The model under review builds one solid part; all positions refer to its coordinate system, in mm. Face numbers are marked on the shaded views. A direction names the side the tool comes from. Coordinates: 2 decimals unless noted, no trailing zeros. Loops run counter-clockwise (first coordinate to the right, second up) from the corner with the lowest first, then second, coordinate; pieces in that order, holes last. Notation, with made-up numbers: (-14.5, 47.25) - (3.5, 47.25) arc R16 ccw to (3.5, 78.25) - close; hole circle Ø6 at (37.5, 15.25). An arc over 180 degrees is marked (long way). Use a Markdown table: item, result. Add a question column.
1) To check wall thickness, follow L1, parallel to X at y = 0, z = 12.6; L2, parallel to X at y = 0, z = 7; L3, parallel to Y at x = -6.4, z = 0.7. State the ranges of each line that lie inside material, in increasing order. Write a range as [from, to].
2) Clearance check with flat-ended pins moving along their axes: pin 1 (2.5 mm diameter, centred on x = -18, y = -0.5, fed in from +Z); pin 2 (3 mm diameter, centred on x = 18.5, y = -1, fed in from +Z); pin 3 (2.5 mm diameter, centred on x = 1, z = 14.5, fed in from +Y). State where each tip first meets the part, or that it passes through.
3) For the marked faces 4, 5 and 6, list the 3-axis set-ups (+Z, -Z, +X, -X, +Y, -Y) from which the entire face can be reached by the end or side of a thin tool; tool diameter is ignored.
4) Add section C-C, the plane z = 11.5. Give the boundary of the cut face in (x, y), and give its area (3 significant figures).
5) The part is to be moulded in two halves that separate along Y. For the marked faces 1, 2 and 3, say which applies: pulls with the +Y half, pulls with the -Y half, needs draft (parallel to the pull), parting line crosses it, or undercut.
6) Add section A-A, the plane y = -14.5. Give the boundary of the cut face in (x, z).
7) Add section D-D, the plane z = 15.25. Give the boundary of the cut face in (x, y), and give its area (3 significant figures).
8) Add section B-B, the plane x = -6.4. Give the number of separate pieces and of enclosed holes in the cut face, and give its area (3 significant figures).
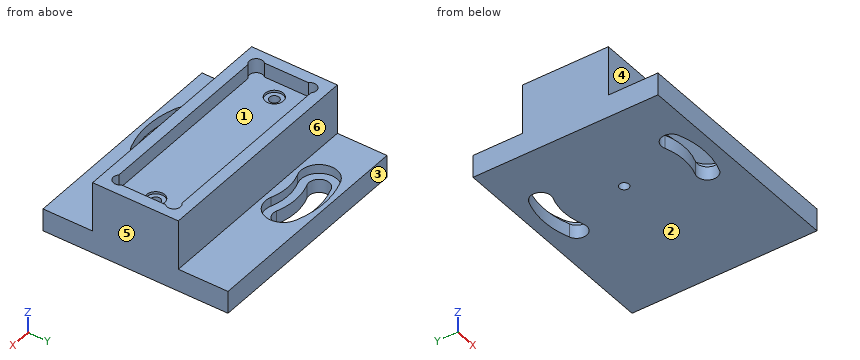
Autodesk Inventor part; units mm, degrees
ref_plane "YZ Plane" through (0, 0, 0) normal (1, 0, 0) x (0, 1, 0)
ref_plane "XZ Plane" through (0, 0, 0) normal (0, 1, 0) x (-1, 0, 0)
ref_plane "XY Plane" through (0, 0, 0) normal (0, 0, 1) x (1, 0, 0)
sketch "Sketch1" plane through (0, 0, 0) normal (0, 0, 1) x (1, 0, 0)
  line L0 (-24.4, -9.5) -> (24.4, -9.5)
  line L1 (24.4, -9.5) -> (24.4, 9.5)
  line L2 (24.4, 9.5) -> (-24.4, 9.5)
  line L3 (-24.4, 9.5) -> (-24.4, -9.5)
  line L4 (-24.4, -9.5) -> (24.4, 9.5) construction
  line L5 (24.4, -9.5) -> (-24.4, 9.5) construction
  point P0 (0, 0)
  dimension "LENGTH" = 48.8
  dimension "WIDTH" = 19
extrude "Extrusion1" add sketch "Sketch1" along normal blind 12.85
sketch "Sketch2" plane through (0, 0, 12.85) normal (0, 0, 1) x (1, 0, 0)
  point P0 (0, 0)
  point P1 (-18.2, 0)
  point P2 (18.2, 0)
  dimension "d11" = 0
  dimension "d12" = 0
  dimension "d13" = 36.4
  dimension "d14" = 18.2
hole "Hole1" at (-18.2, 0, 12.85) at (18.2, 0, 12.85) direction (0, 0, -1) diameter 2.1565 depth 8.87
sketch "Sketch3" plane through (0, 0, 12.85) normal (0, 0, 1) x (1, 0, 0)
  point P0 (0, 0)
  point P1 (0, 0)
  dimension "d22" = 0
  dimension "d23" = 0
hole "Hole2" [suppressed]
sketch "Sketch4" plane through (0, 0, 0) normal (0, 0, -1) x (-1, 0, 0)
  line L0 (5.5, 0) -> (4.5, 0) construction
  line L1 (5.5, 1.05) -> (4.5, 1.05)
  line L2 (4.5, -1.05) -> (5.5, -1.05)
  arc A0 (5.5, -1.05) -> (5.5, 1.05) centre (5.5, 0) ccw
  arc A1 (4.5, 1.05) -> (4.5, -1.05) centre (4.5, 0) ccw
  point P0 (0, 0)
  point P1 (-5, 0)
  point P2 (5, 0)
  dimension "d24" = 1
  dimension "d25" = 0
  dimension "d26" = 0
  dimension "d27" = 10
  dimension "d28" = 5
  dimension "d29" = 1.05
hole "Hole3" [suppressed]
extrude "Extrusion2" [suppressed]
sketch "Sketch5" plane through (0, 0, 0) normal (0, 0, 1) x (1, 0, 0)
  line L0 (-24.4, -20.5) -> (24.4, -20.5)
  line L1 (24.4, -20.5) -> (24.4, 20.5)
  line L2 (24.4, 20.5) -> (-24.4, 20.5)
  line L3 (-24.4, 20.5) -> (-24.4, -20.5)
  line L4 (-24.4, -20.5) -> (24.4, 20.5) construction
  line L5 (24.4, -20.5) -> (-24.4, 20.5) construction
  point P0 (0, 0)
  dimension "d39" = 48.8
  dimension "d40" = 41
extrude "Extrusion3" add sketch "Sketch5" along normal blind 5
sketch "Sketch7" plane through (0, 0, 12.85) normal (0, 0, 1) x (1, 0, 0)
  circle A0 centre (18.2, 0) radius 1.0782
  circle A1 centre (-18.2, 0) radius 1.0782
  point P0 (0, 0)
  dimension "d54" = 0
  dimension "d55" = 0
  dimension "d56" = 0
  dimension "d57" = 0
hole "Hole5" at (18.2, 0, 12.85) at (-18.2, 0, 12.85) direction (0, 0, -1) diameter 4 depth 0.5
sketch "Sketch8" plane through (0, 0, 0) normal (0, 0, -1) x (-1, 0, 0)
  line L0 (0, 5.5) -> (0, 4.5) construction
  line L1 (-1.05, 5.5) -> (-1.05, 4.5)
  line L2 (1.05, 4.5) -> (1.05, 5.5)
  arc A0 (1.05, 5.5) -> (-1.05, 5.5) centre (0, 5.5) ccw
  arc A1 (-1.05, 4.5) -> (1.05, 4.5) centre (0, 4.5) ccw
  point P0 (0, 0)
  point P1 (0, -5)
  point P2 (0, 5)
  dimension "d77" = 1
  dimension "d78" = 1.05
  dimension "d79" = 10
  dimension "d80" = 0
  dimension "d81" = 0
  dimension "d82" = 5
hole "Hole6" [suppressed]
extrude "Extrusion4" [suppressed]
sketch "Sketch10" plane through (0, 0, 12.85) normal (0, 0, 1) x (1, 0, 0)
  line L0 (-24.4, -9.5) -> (24.4, -9.5)
  line L1 (24.4, -9.5) -> (24.4, 9.5)
  line L2 (24.4, 9.5) -> (-24.4, 9.5)
  line L3 (-24.4, 9.5) -> (-24.4, -9.5)
  line L4 (-24.4, -9.5) -> (24.4, 9.5) construction
  line L5 (24.4, -9.5) -> (-24.4, 9.5) construction
  line L6 (21.9, -7) -> (-21.9, -7)
  line L7 (-21.9, -7) -> (-21.9, 7)
  line L8 (-21.9, 7) -> (21.9, 7)
  line L9 (21.9, 7) -> (21.9, -7)
  line L10 (21.9, -7) -> (-21.9, 7) construction
  line L11 (-21.9, -7) -> (21.9, 7) construction
  circle A0 centre (-20.8393, 5.9393) radius 1.5
  circle A1 centre (-20.8393, -5.9393) radius 1.5
  circle A2 centre (20.8393, 5.9393) radius 1.5
  circle A3 centre (20.8393, -5.9393) radius 1.5
  line L12 (20.8393, 5.9393) -> (21.9, 7)
  line L13 (21.9, -7) -> (20.8393, -5.9393)
  line L14 (-20.8393, 5.9393) -> (-21.9, 7)
  line L15 (-20.8393, -5.9393) -> (-21.9, -7)
  point P0 (0, 0)
  point P1 (21.9, -4.8787)
  point P2 (19.7787, -7)
  point P3 (-19.7787, -7)
  point P4 (-21.9, -4.8787)
  point P5 (-21.9, 4.8787)
  point P6 (-19.7787, 7)
  point P7 (19.7787, 7)
  point P8 (21.9, 4.8787)
  dimension "d106" = 3
  dimension "d110" = 3
  dimension "d111" = 3
  dimension "d112" = 3
  dimension "d97" = 48.8
  dimension "d98" = 19
  dimension "d99" = 43.8
  dimension "d100" = 14
  dimension "d107" = 45
  dimension "d108" = 45
  dimension "d109" = 45
extrude "Extrusion6" add sketch "Sketch10" along normal blind 3.2
chamfer "Chamfer5" [suppressed]
sketch "Sketch12" plane through (0, 0, 5) normal (0, 0, 1) x (1, 0, 0)
  arc A0 (7.9961, 15.4962) -> (-8.004, 14.5013) centre (9.4196, -136.543) ccw construction
  arc A1 (7.9587, 19.496) -> (-8.4624, 18.4749) centre (9.4196, -136.543) ccw
  arc A2 (8.0336, 11.4964) -> (-7.5457, 10.5276) centre (9.4196, -136.543) ccw
  arc A3 (8.0336, 11.4964) -> (7.9587, 19.496) centre (7.9961, 15.4962) ccw
  arc A4 (-8.4624, 18.4749) -> (-7.5457, 10.5276) centre (-8.004, 14.5013) ccw
  line L0 (24.4, 2.961) -> (24.4, -2.961)
  line L1 (24.4, 0) -> (-24.4, 0)
  line L2 (-24.4, 8.5) -> (-24.4, -8.5)
  arc A5 (7.9961, 15.4962) -> (-8.004, 14.5013) centre (9.4196, -136.543) ccw construction
  arc A6 (7.9751, 17.7461) -> (-8.2619, 16.7364) centre (9.4196, -136.543) ccw
  arc A7 (8.0172, 13.2463) -> (-7.7462, 12.2661) centre (9.4196, -136.543) ccw
  arc A8 (8.0172, 13.2463) -> (7.9751, 17.7461) centre (7.9961, 15.4962) ccw
  arc A9 (-8.2619, 16.7364) -> (-7.7462, 12.2661) centre (-8.004, 14.5013) ccw
  arc A10 (-8.004, -14.5013) -> (7.9961, -15.4962) centre (9.4196, 136.543) ccw construction
  arc A11 (-8.4624, -18.4749) -> (7.9587, -19.496) centre (9.4196, 136.543) ccw
  arc A12 (-7.5457, -10.5276) -> (8.0336, -11.4964) centre (9.4196, 136.543) ccw
  arc A13 (7.9587, -19.496) -> (8.0336, -11.4964) centre (7.9961, -15.4962) ccw
  arc A14 (-7.5457, -10.5276) -> (-8.4624, -18.4749) centre (-8.004, -14.5013) ccw
  arc A15 (-8.004, -14.5013) -> (7.9961, -15.4962) centre (9.4196, 136.543) ccw construction
  arc A16 (-8.2619, -16.7364) -> (7.9751, -17.7461) centre (9.4196, 136.543) ccw
  arc A17 (-7.7462, -12.2661) -> (8.0172, -13.2463) centre (9.4196, 136.543) ccw
  arc A18 (7.9751, -17.7461) -> (8.0172, -13.2463) centre (7.9961, -15.4962) ccw
  arc A19 (-7.7462, -12.2661) -> (-8.2619, -16.7364) centre (-8.004, -14.5013) ccw
  point P0 (0, 0)
  point P1 (-8.004, 12.753)
  point P2 (7.9961, 17.2527)
  point P3 (-6.4165, 14.3405)
  point P4 (9.5836, 18.8402)
  point P5 (-8.004, -12.753)
  point P6 (7.9961, -17.2527)
  point P7 (9.5836, -18.8402)
  point P8 (-6.4165, -14.3405)
  dimension "d118" = 8
  dimension "d122" = 4.5
extrude "Extrusion12" [suppressed]
extrude "Extrusion13" [suppressed]
sketch "Sketch14" plane through (0, 0, 0) normal (0, 0, -1) x (-1, 0, 0)
  point P0 (0, 0)
  point P1 (6.4, 0)
hole "Hole7" at (-6.4, 0, 0) direction (0, 0, 1) diameter 2.1 depth 2.1
sketch "Sketch15" plane through (0, 0, 0) normal (0, 0, -1) x (-1, 0, 0)
  circle A0 centre (6.4, 0) radius 1.05
  circle A1 centre (6.4, 0) radius 19.5
  circle A2 centre (6.4, 0) radius 11.5
  circle A3 centre (6.4, 0) radius 17.75
  circle A4 centre (6.4, 0) radius 13.25
  line L0 (-24.4, 9.5) -> (24.4, 9.5)
  line L1 (24.4, 9.5) -> (-24.4, 9.5)
  line L2 (-24.4, -20.5) -> (-24.4, 20.5)
  line L3 (24.4, -9.5) -> (-24.4, -9.5)
  line L4 (24.4, -9.5) -> (-24.4, -9.5)
  arc A5 (9.3371, 17.5053) -> (5.1369, 17.705) centre (6.4, 0) ccw
  arc A6 (8.5925, 13.0673) -> (5.4572, 13.2164) centre (6.4, 0) ccw
  arc A7 (13.9857, 17.9641) -> (-1.4292, 17.8592) centre (6.4, 0) ccw
  arc A8 (10.8736, 10.5942) -> (1.7828, 10.5324) centre (6.4, 0) ccw
  arc A9 (11.8707, 14.5025) -> (0.9294, 14.5025) centre (6.4, 0) ccw construction
  arc A10 (13.2825, 18.2451) -> (-0.4824, 18.2451) centre (6.4, 0) ccw
  arc A11 (10.4589, 10.7599) -> (2.3412, 10.7599) centre (6.4, 0) ccw
  arc A12 (10.4589, 10.7599) -> (13.2825, 18.2451) centre (11.8707, 14.5025) ccw
  arc A13 (-0.4824, 18.2451) -> (2.3412, 10.7599) centre (0.9294, 14.5025) ccw
  arc A14 (11.8707, 14.5025) -> (0.9294, 14.5025) centre (6.4, 0) ccw construction
  arc A15 (12.6648, 16.6077) -> (0.1352, 16.6077) centre (6.4, 0) ccw
  arc A16 (11.0766, 12.3973) -> (1.7235, 12.3973) centre (6.4, 0) ccw
  arc A17 (11.0766, 12.3973) -> (12.6648, 16.6077) centre (11.8707, 14.5025) ccw
  arc A18 (0.1352, 16.6077) -> (1.7235, 12.3973) centre (0.9294, 14.5025) ccw
  line L5 (24.4, 9.5) -> (24.4, -9.5)
  line L6 (24.4, 0) -> (-24.4, 0)
  arc A19 (5.1369, -17.705) -> (9.3371, -17.5053) centre (6.4, 0) ccw
  arc A20 (5.4572, -13.2164) -> (8.5925, -13.0673) centre (6.4, 0) ccw
  arc A21 (-1.4292, -17.8592) -> (13.9857, -17.9641) centre (6.4, 0) ccw
  arc A22 (1.7828, -10.5324) -> (10.8736, -10.5942) centre (6.4, 0) ccw
  arc A23 (0.9294, -14.5025) -> (11.8707, -14.5025) centre (6.4, 0) ccw construction
  arc A24 (-0.4824, -18.2451) -> (13.2825, -18.2451) centre (6.4, 0) ccw
  arc A25 (2.3412, -10.7599) -> (10.4589, -10.7599) centre (6.4, 0) ccw
  arc A26 (13.2825, -18.2451) -> (10.4589, -10.7599) centre (11.8707, -14.5025) ccw
  arc A27 (2.3412, -10.7599) -> (-0.4824, -18.2451) centre (0.9294, -14.5025) ccw
  arc A28 (0.9294, -14.5025) -> (11.8707, -14.5025) centre (6.4, 0) ccw construction
  arc A29 (0.1352, -16.6077) -> (12.6648, -16.6077) centre (6.4, 0) ccw
  arc A30 (1.7235, -12.3973) -> (11.0766, -12.3973) centre (6.4, 0) ccw
  arc A31 (12.6648, -16.6077) -> (11.0766, -12.3973) centre (11.8707, -14.5025) ccw
  arc A32 (1.7235, -12.3973) -> (0.1352, -16.6077) centre (0.9294, -14.5025) ccw
  point P0 (0, 0)
  point P1 (-24.4, -19.5)
  point P2 (-24.4, 19.5)
  point P3 (24.4, 8.5)
  point P4 (24.4, -8.5)
  point P5 (6.4, 15.5)
  point P6 (6.4, -15.5)
  dimension "d140" = 39
  dimension "d141" = 23
  dimension "d142" = 35.5
  dimension "d143" = 26.5
  dimension "d147" = 8
  dimension "d148" = 4.5
sketch "Sketch17" plane through (0, 0, 5) normal (0, 0, 1) x (1, 0, 0)
  circle A0 centre (-6.4, 0) radius 1.05
  arc A1 (-11.8725, -14.4958) -> (-0.9318, -14.4974) centre (-6.4, 0) ccw construction
  arc A2 (-12.6672, -16.6008) -> (-0.1378, -16.6026) centre (-6.4, 0) ccw
  arc A3 (-11.0779, -12.3908) -> (-1.7259, -12.3922) centre (-6.4, 0) ccw
  arc A4 (-11.0779, -12.3908) -> (-12.6672, -16.6008) centre (-11.8725, -14.4958) ccw
  arc A5 (-0.1378, -16.6026) -> (-1.7259, -12.3922) centre (-0.9318, -14.4974) ccw
  arc A6 (-11.8725, -14.4958) -> (-0.9318, -14.4974) centre (-6.4, 0) ccw construction
  arc A7 (-13.2853, -18.238) -> (0.4798, -18.24) centre (-6.4, 0) ccw
  arc A8 (-10.4598, -10.7536) -> (-2.3435, -10.7548) centre (-6.4, 0) ccw
  arc A9 (-10.4598, -10.7536) -> (-13.2853, -18.238) centre (-11.8725, -14.4958) ccw
  arc A10 (0.4798, -18.24) -> (-2.3435, -10.7548) centre (-0.9318, -14.4974) ccw
  line L0 (-24.1444, 0) -> (24.3913, 0)
  line L1 (24.3913, 0) -> (-24.1444, 0)
  arc A11 (-0.9318, 14.4974) -> (-11.8725, 14.4958) centre (-6.4, 0) ccw construction
  arc A12 (-0.1378, 16.6026) -> (-12.6672, 16.6008) centre (-6.4, 0) ccw
  arc A13 (-1.7259, 12.3922) -> (-11.0779, 12.3908) centre (-6.4, 0) ccw
  arc A14 (-12.6672, 16.6008) -> (-11.0779, 12.3908) centre (-11.8725, 14.4958) ccw
  arc A15 (-1.7259, 12.3922) -> (-0.1378, 16.6026) centre (-0.9318, 14.4974) ccw
  arc A16 (-0.9318, 14.4974) -> (-11.8725, 14.4958) centre (-6.4, 0) ccw construction
  arc A17 (0.4798, 18.24) -> (-13.2853, 18.238) centre (-6.4, 0) ccw
  arc A18 (-2.3435, 10.7548) -> (-10.4598, 10.7536) centre (-6.4, 0) ccw
  arc A19 (-13.2853, 18.238) -> (-10.4598, 10.7536) centre (-11.8725, 14.4958) ccw
  arc A20 (-2.3435, 10.7548) -> (0.4798, 18.24) centre (-0.9318, 14.4974) ccw
  point P0 (0, 0)
  point P1 (-0.9324, -14.4958)
  point P2 (-0.9324, 14.4958)
  dimension "d149" = 4.5
  dimension "d150" = 8
extrude "Extrusion14" cut sketch "Sketch17" against normal through all contours A4 A3 A5 A2 | A15 A13 A14 A12
extrude "Extrusion15" cut sketch "Sketch17" against normal blind 2 contours A9 A8 A10 A7 | A20 A18 A19 A17
equation "\"d2\" = BEAM_HEIGHT - APERTURE_HEIGHT"
equation "\"d39\" = LENGTH"
equation "\"d106\" = d110"
equation "\"d111\" = d110"
equation "\"d112\" = d110"
equation "\"d97\" = LENGTH"
equation "\"d98\" = WIDTH"
equation "\"BEAM_HEIGHT\" = 19.05"
equation "\"APERTURE_HEIGHT\" = 6.2"
properties part number "ADAPTER_AOM-brimrose"
From the geometry:
| question | item | result |
|---|---|---|
| 1 | L1 | x = [-24.4, -20.2], [-16.2, 16.2], [20.2, 24.4] |
| 1 | L2 | x = [-24.4, -19.28], [-17.12, 17.12], [19.28, 24.4] |
| 1 | L3 | y = [-20.5, -17.74], [-13.24, -1.05], [1.05, 13.24], [17.74, 20.5] |
| 2 | pin 1 | stops at z = 12.35 |
| 2 | pin 2 | stops at z = 12.85 |
| 2 | pin 3 | stops at y = 9.5 |
| 3 | face 4 | +Z, +X, -X, -Y |
| 3 | face 5 | +Z, -Z, +X, +Y, -Y |
| 3 | face 6 | +Z, +X, -X, +Y |
| 4 | outline | (-24.4, -9.5) - (24.4, -9.5) - (24.4, 9.5) - (-24.4, 9.5) - close; hole circle Ø2.16 at (-18.2, 0); hole circle Ø2.16 at (18.2, 0) |
| 4 | area | 920 mm^2 |
| 5 | face 1 | undercut |
| 5 | face 2 | needs draft |
| 5 | face 3 | pulls with the +Y half |
| 6 | outline | (-24.4, 0) - (-14.12, 0) - (-14.12, 3) - (-15.87, 3) - (-15.87, 5) - (-24.4, 5) - close; (1.32, 0) - (24.4, 0) - (24.4, 5) - (3.07, 5) - (3.07, 3) - (1.32, 3) - close |
| 7 | outline | (-24.4, -9.5) - (24.4, -9.5) - (24.4, 9.5) - (-24.4, 9.5) - close; hole (-21.9, -4.88) arc R1.5 ccw to (-19.78, -7) - (19.78, -7) arc R1.5 ccw to (21.9, -4.88) - (21.9, 4.88) arc R1.5 ccw to (19.78, 7) - (-19.78, 7) arc R1.5 ccw to (-21.9, 4.88) - close |
| 7 | area | 309 mm^2 |
| 8 | separate pieces | 3 |
| 8 | enclosed holes | 0 |
| 8 | area | 307 mm^2 |
